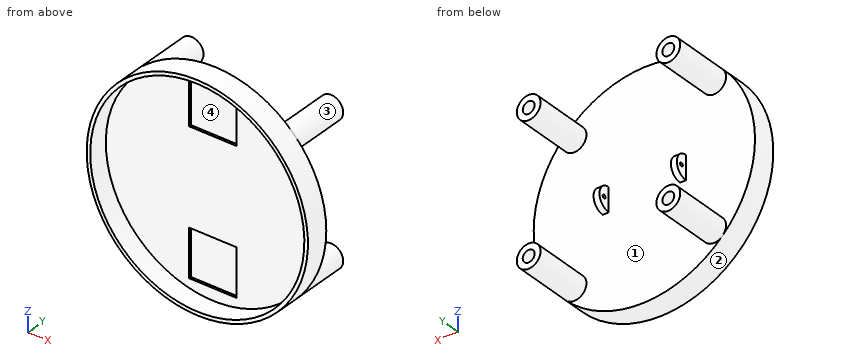
from build123d import *

# Parameters (mm, degrees)
SKETCH1_R           = 93
BOSS_EXTRUDE1_DEPTH = 20
SHELL1_T            = -3
SKETCH2_W           = 5
SKETCH2_H           = 10
REVOLVE1_ANGLE      = 180
SKETCH7_R           = 1.5
CUT_EXTRUDE1_DEPTH  = 10
SKETCH8_W           = 40
SKETCH8_H           = 40
CUT_EXTRUDE2_DEPTH  = 2
SKETCH9_R           = 10
BOSS_EXTRUDE2_DEPTH = 50
SKETCH10_R          = 5
CUT_EXTRUDE3_DEPTH  = 20
CIRPATTERN1_COUNT   = 4


with BuildPart() as part:
    # Sketch1 → Boss-Extrude1 (new body)
    with BuildSketch(Plane(origin=(0, 0, 0), x_dir=(1, 0, 0), z_dir=(0, 1, 0))):
        with Locations(Location((0, 0, 0), (0, 0, 270))):
            Circle(SKETCH1_R)
    extrude(amount=BOSS_EXTRUDE1_DEPTH)

    # Shell1
    shell1_openings = [part.faces().sort_by_distance(p)[0] for p in [
        (0, 0, 0),
    ]]
    offset(amount=SHELL1_T, openings=shell1_openings, kind=Kind.INTERSECTION)

    # Sketch2 → Revolve1 (revolve)
    with BuildSketch(Plane(origin=(0, 20, 0), x_dir=(1, 0, 0), z_dir=(0, 1, 0))):
        with Locations((-32.5, 5)):
            Rectangle(SKETCH2_W, SKETCH2_H)
    revolve1 = revolve(axis=Axis((0, 20, 0), (1, 0, 0)), revolution_arc=REVOLVE1_ANGLE)

    # Sketch7 → Cut-Extrude1 (cut)
    with BuildSketch(Plane.ZY.offset(35)):
        with Locations((0, 25)):
            Circle(SKETCH7_R)
    cut_extrude1 = extrude(amount=-CUT_EXTRUDE1_DEPTH, mode=Mode.SUBTRACT)

    # Mirror1: Revolve1, Cut-Extrude1 across plane
    add(revolve1.mirror(Plane(origin=(0, 0, 0), x_dir=(0, 0, 1), z_dir=(1, 0, 0))))
    add(cut_extrude1.mirror(Plane(origin=(0, 0, 0), x_dir=(0, 0, 1), z_dir=(1, 0, 0))), mode=Mode.SUBTRACT)

    # Sketch8 → Cut-Extrude2 (cut)
    with BuildSketch(Plane.XZ.offset(-17)):
        with Locations((0, 60)):
            Rectangle(SKETCH8_W, SKETCH8_H)
    cut_extrude2 = extrude(amount=-CUT_EXTRUDE2_DEPTH, mode=Mode.SUBTRACT)

    # Mirror2: Cut-Extrude2 across plane
    add(cut_extrude2.mirror(Plane.XY), mode=Mode.SUBTRACT)

    # Sketch9 → Boss-Extrude2 (add)
    with BuildSketch(Plane(origin=(0, 20, 0), x_dir=(1, 0, 0), z_dir=(0, 1, 0))):
        with Locations(Location((-58.689862838, 58.689862838, 0), (0, 0, 135))):
            Circle(SKETCH9_R)
    boss_extrude2 = extrude(amount=BOSS_EXTRUDE2_DEPTH)

    # Sketch10 → Cut-Extrude3 (cut)
    with BuildSketch(Plane(origin=(0, 70, 0), x_dir=(1, 0, 0), z_dir=(0, 1, 0))):
        with Locations(Location((-58.689862838, 58.689862838, 0), (0, 0, 270))):
            Circle(SKETCH10_R)
    cut_extrude3 = extrude(amount=-CUT_EXTRUDE3_DEPTH, mode=Mode.SUBTRACT)

    # CirPattern1: Boss-Extrude2, Cut-Extrude3 ×4 about axis
    cirpattern1_axis = Axis((0, 0, 0), (0, 1, 0))
    add([boss_extrude2.rotate(cirpattern1_axis, i * 360 / CIRPATTERN1_COUNT) for i in range(1, CIRPATTERN1_COUNT)])
    add([cut_extrude3.rotate(cirpattern1_axis, i * 360 / CIRPATTERN1_COUNT) for i in range(1, CIRPATTERN1_COUNT)], mode=Mode.SUBTRACT)


solid = part.part
Read the model definition and answer for the solid it produces. Units are mm, in the model's axes. Face numbers are marked on the shaded views. A direction names the side the tool comes from. Round coordinates to 2 decimals unless told otherwise and drop trailing zeros. Loops run counter-clockwise (first coordinate to the right, second up) from the corner with the lowest first, then second, coordinate; pieces in that order, holes last.
Q1. Section B-B on x = 0 is taken. Write down the section's boundary in (y, z).
Q2. Which of the six approach directions +Z, -Z, +X, -X, +Y, -Y give full straight-line access (tool end or side, diameter ignored) to the marked faces 3 and 4?
Q3. Section C-C on z = 43 is taken. Write down the section's boundary in (x, y).
Q4. Section A-A on y = 54 is taken. Write down the section's boundary in (x, z), and give its area (3 significant figures).
Q5. Section D-D on y = 6.5 is taken. Write down the section's boundary in (x, z), and give its area (3 significant figures).
Q6. Consider probe 1 along Z at (x, y) = (0, 8); probe 2 along Y at (x, z) = (33.15, 0). Determine where each line is inside the solid, lowest interval first.
Q7. Determine the mould class of the marked faces 1 and 2 for opening direction X: released by +X, released by -X, zero draft, split by the parting line, or undercut.
Q8. Each of these flat-tipped pins is pushed along its axis until it touches: pin 1 (1.6 mm diameter, centred on x = -6, y = 18, fed in from +Z); pin 2 (3.5 mm diameter, centred on y = 25, z = 0, fed in from -X); pin 3 (8 mm diameter, centred on x = -65.5, z = 42.5, fed in from -Y). Where does it stop, or does it pass through?
Output:
1. outline: (0, -93) - (20, -93) - (20, 93) - (0, 93) - (0, 90) - (17, 90) - (17, 80) - (19, 80) - (19, 40) - (17, 40) - (17, -40) - (19, -40) - (19, -80) - (17, -80) - (17, -90) - (0, -90) - close
2. face 3: +Y
2. face 4: -Y
3. outline: (-82.46, 0) - (-79.06, 0) - (-79.06, 17) - (-20, 17) - (-20, 19) - (20, 19) - (20, 17) - (79.06, 17) - (79.06, 0) - (82.46, 0) - (82.46, 20) - (-82.46, 20) - close
4. outline: circle Ø20 at (-58.69, -58.69); circle Ø20 at (-58.69, 58.69); circle Ø20 at (58.69, -58.69); circle Ø20 at (58.69, 58.69); hole circle Ø10 at (-58.69, -58.69); hole circle Ø10 at (-58.69, 58.69); hole circle Ø10 at (58.69, -58.69); hole circle Ø10 at (58.69, 58.69)
4. area: 942 mm2
5. outline: circle Ø186 at (0, 0); hole circle Ø180 at (0, 0)
5. area: 1,720 mm2
6. probe 1: z = -93 to -90, 90 to 93
6. probe 2: y = 17 to 23.5, 26.5 to 30
7. face 1: undercut
7. face 2: split by the parting line
8. pin 1: stops at z = 92.85
8. pin 2: stops at x = -35
8. pin 3: stops at y = 17
